Input: part model. Units: mm. Frame: model coordinates. A direction names the side the tool comes from. Coordinates: 2 decimals unless noted, no trailing zeros. Loops run counter-clockwise (first coordinate to the right, second up) from the corner with the lowest first, then second, coordinate; pieces in that order, holes last.
(1) Section A-A, the plane z = 21. Return loops of the section in (x, y).
(2) Line query: L1, parallel to Z at x = 1.25, y = -5; L2, parallel to X at y = -1, z = 23; L3, parallel to X at y = -0.5, z = 14. Output: solid intervals per line, ascending.
(3) Set-up query: faces 1 (the face through (-0.867, -3.905, 17.825)), 2 (the face through (-3.343, 5.82, 0.103)). Return all of +Z, -Z, +X, -X, +Y, -Y with unobstructed straight access to the full face (end or side cutting, diameter ignored); none if empty.
(4) Contact query for flat-ended pins moving along their axis: P1, Ø6, axis at y = -1, z = 10, coming from the -X side; P2, Ø5, axis at x = -2, y = 2.5, coming from the -Z side; P3, Ø3, axis at x = 5, y = 3.5, coming from the +Z side; P4, Ø1, axis at x = -0.5, z = 22.5, coming from the -Y side. Output: stop coordinate, or through.
```python
from build123d import *

# Parameters (mm, degrees)
PAD008_DEPTH = 5.5
SKETCH029_R  = 4
PAD009_DEPTH = 25


with BuildPart() as part:
    # Sketch028 → Pad008 (new body)
    with BuildSketch(Plane.XY):
        Polygon((7.5055534995, 0), (3.7527767497, 6.5), (-3.7527767497, 6.5), (-7.5055534995, 0), (-3.7527767497, -6.5), (3.7527767497, -6.5), align=None)
    extrude(amount=PAD008_DEPTH)

    # Sketch029 (on Face8 of Pad008) → Pad009 (join)
    with BuildSketch(Plane.XY.offset(5.5)):
        Circle(SKETCH029_R)
    extrude(amount=PAD009_DEPTH)

    # Sketch030 → Groove001 (revolve, cut)
    with BuildSketch(Plane.XZ):
        Polygon((4, 30.5), (3.5, 30.5), (4, 31), align=None)
        Polygon((7.5055534995, 5.5), (6.5055534995, 5.5), (7.5055534995, 5), align=None)
        Polygon((7.5055534995, 0), (6.5055534995, 0), (7.5055534995, 0.5), align=None)
    revolve(axis=Axis((0, 0, 0), (0, 0, 1)), mode=Mode.SUBTRACT)


solid = part.part
```
Report:
1. outline: circle Ø8 at (0, 0)
2. L1: z = 0 to 5.5
2. L2: x = -3.87 to 3.87
2. L3: x = -3.97 to 3.97
3. face 1: +Z
3. face 2: -Z, -X, +Y
4. P1: stops at x = -4
4. P2: stops at z = 0
4. P3: stops at z = 5.5
4. P4: stops at y = -4
